For this review, take the finished solid that the model builds, in its own axes (mm). A direction names the side the tool comes from. Round coordinates to 2 decimals unless told otherwise and drop trailing zeros. Order: outer loops, then holes, each group sorted by start corner. A loop starts at its lowest first (then second) coordinate and runs counter-clockwise, first axis right, second up. Notation, with made-up numbers: (-21.75, 44) - (-7.75, 44) arc R11 cw to (-7.75, 57) - close; hole circle Ø10 at (52.25, 86). An arc over 180 degrees is marked (long way). One line per item, written item: value.
```python
from build123d import *

# Parameters (mm, degrees)
AUFSATZ_LINEAR_AUSTRAGEN1_DEPTH = 1.5
SCHNITT_LINEAR_AUSTRAGEN1_REACH = 159.472
SKIZZE2_R                       = 1.3
SKIZZE2_R_2                     = 1
SCHNITT_LINEAR_AUSTRAGEN2_REACH = 159.472
SKIZZE3_W                       = 27
SKIZZE3_H                       = 17.5
SKIZZE4_R                       = 2.5
SKIZZE4_R_2                     = 1.3
AUFSATZ_LINEAR_AUSTRAGEN2_DEPTH = 3
VERRUNDUNG1_R                   = 2
SCHNITT_LINEAR_AUSTRAGEN3_REACH = 159.494
SKIZZE5_W                       = 71.8
SKIZZE5_H                       = 18
VERRUNDUNG2_R                   = 2
SCHNITT_LINEAR_AUSTRAGEN4_REACH = 159.494
SKIZZE6_W                       = 6
SKIZZE6_H                       = 2


with BuildPart() as part:
    # Skizze1 → Aufsatz-Linear austragen1 (new body)
    with BuildSketch(Plane.XY):
        with BuildLine():
            Line((8.4, 0), (113.4, 0))
            ThreePointArc((113.4, 0), (119.339696962, 2.460303038), (121.8, 8.4))
            Line((121.8, 8.4), (121.8, 91.4))
            ThreePointArc((121.8, 91.4), (119.339696962, 97.339696962), (113.4, 99.8))
            Line((113.4, 99.8), (8.4, 99.8))
            ThreePointArc((8.4, 99.8), (2.460303038, 97.339696962), (0, 91.4))
            Line((0, 91.4), (0, 8.4))
            ThreePointArc((0, 8.4), (2.460303038, 2.460303038), (8.4, 0))
        make_face()
    extrude(amount=AUFSATZ_LINEAR_AUSTRAGEN1_DEPTH)

    # Skizze2 → Schnitt-Linear austragen1 (cut, up to next)
    with BuildSketch(Plane.XY.offset(1.5), mode=Mode.PRIVATE) as schnitt_linear_austragen1_sk1:
        with Locations((45.8, 54.2)):
            Circle(SKIZZE2_R)
    schnitt_linear_austragen1_tool1 = extrude(schnitt_linear_austragen1_sk1.sketch, amount=-SCHNITT_LINEAR_AUSTRAGEN1_REACH, mode=Mode.PRIVATE) & part.part
    # Skizze2 → Schnitt-Linear austragen1 (cut, up to next)
    with BuildSketch(Plane.XY.offset(1.5), mode=Mode.PRIVATE) as schnitt_linear_austragen1_sk2:
        with Locations((45.8, 5.2)):
            Circle(SKIZZE2_R)
    schnitt_linear_austragen1_tool2 = extrude(schnitt_linear_austragen1_sk2.sketch, amount=-SCHNITT_LINEAR_AUSTRAGEN1_REACH, mode=Mode.PRIVATE) & part.part
    # Skizze2 → Schnitt-Linear austragen1 (cut, up to next)
    with BuildSketch(Plane.XY.offset(1.5), mode=Mode.PRIVATE) as schnitt_linear_austragen1_sk3:
        with Locations((103.8, 54.2)):
            Circle(SKIZZE2_R)
    schnitt_linear_austragen1_tool3 = extrude(schnitt_linear_austragen1_sk3.sketch, amount=-SCHNITT_LINEAR_AUSTRAGEN1_REACH, mode=Mode.PRIVATE) & part.part
    # Skizze2 → Schnitt-Linear austragen1 (cut, up to next)
    with BuildSketch(Plane.XY.offset(1.5), mode=Mode.PRIVATE) as schnitt_linear_austragen1_sk4:
        with Locations((103.8, 5.2)):
            Circle(SKIZZE2_R)
    schnitt_linear_austragen1_tool4 = extrude(schnitt_linear_austragen1_sk4.sketch, amount=-SCHNITT_LINEAR_AUSTRAGEN1_REACH, mode=Mode.PRIVATE) & part.part
    # Skizze2 → Schnitt-Linear austragen1 (cut, up to next)
    with BuildSketch(Plane.XY.offset(1.5), mode=Mode.PRIVATE) as schnitt_linear_austragen1_sk5:
        with Locations((5.4, 94.4)):
            Circle(SKIZZE2_R_2)
    schnitt_linear_austragen1_tool5 = extrude(schnitt_linear_austragen1_sk5.sketch, amount=-SCHNITT_LINEAR_AUSTRAGEN1_REACH, mode=Mode.PRIVATE) & part.part
    # Skizze2 → Schnitt-Linear austragen1 (cut, up to next)
    with BuildSketch(Plane.XY.offset(1.5), mode=Mode.PRIVATE) as schnitt_linear_austragen1_sk6:
        with Locations((116.4, 94.4)):
            Circle(SKIZZE2_R_2)
    schnitt_linear_austragen1_tool6 = extrude(schnitt_linear_austragen1_sk6.sketch, amount=-SCHNITT_LINEAR_AUSTRAGEN1_REACH, mode=Mode.PRIVATE) & part.part
    # Skizze2 → Schnitt-Linear austragen1 (cut, up to next)
    with BuildSketch(Plane.XY.offset(1.5), mode=Mode.PRIVATE) as schnitt_linear_austragen1_sk7:
        with Locations((116.4, 5.4)):
            Circle(SKIZZE2_R_2)
    schnitt_linear_austragen1_tool7 = extrude(schnitt_linear_austragen1_sk7.sketch, amount=-SCHNITT_LINEAR_AUSTRAGEN1_REACH, mode=Mode.PRIVATE) & part.part
    # Skizze2 → Schnitt-Linear austragen1 (cut, up to next)
    with BuildSketch(Plane.XY.offset(1.5), mode=Mode.PRIVATE) as schnitt_linear_austragen1_sk8:
        with Locations((5.4, 5.4)):
            Circle(SKIZZE2_R_2)
    schnitt_linear_austragen1_tool8 = extrude(schnitt_linear_austragen1_sk8.sketch, amount=-SCHNITT_LINEAR_AUSTRAGEN1_REACH, mode=Mode.PRIVATE) & part.part
    add(schnitt_linear_austragen1_tool1.solids().sort_by_distance((45.8, 54.2, 1.5))[0], mode=Mode.SUBTRACT)
    add(schnitt_linear_austragen1_tool2.solids().sort_by_distance((45.8, 5.2, 1.5))[0], mode=Mode.SUBTRACT)
    add(schnitt_linear_austragen1_tool3.solids().sort_by_distance((103.8, 54.2, 1.5))[0], mode=Mode.SUBTRACT)
    add(schnitt_linear_austragen1_tool4.solids().sort_by_distance((103.8, 5.2, 1.5))[0], mode=Mode.SUBTRACT)
    add(schnitt_linear_austragen1_tool5.solids().sort_by_distance((5.4, 94.4, 1.5))[0], mode=Mode.SUBTRACT)
    add(schnitt_linear_austragen1_tool6.solids().sort_by_distance((116.4, 94.4, 1.5))[0], mode=Mode.SUBTRACT)
    add(schnitt_linear_austragen1_tool7.solids().sort_by_distance((116.4, 5.4, 1.5))[0], mode=Mode.SUBTRACT)
    add(schnitt_linear_austragen1_tool8.solids().sort_by_distance((5.4, 5.4, 1.5))[0], mode=Mode.SUBTRACT)

    # Skizze3 → Schnitt-Linear austragen2 (cut, up to next)
    with BuildSketch(Plane.XY.offset(1.5), mode=Mode.PRIVATE) as schnitt_linear_austragen2_sk1:
        with Locations((100.3, 81.05)):
            Rectangle(SKIZZE3_W, SKIZZE3_H)
    schnitt_linear_austragen2_tool1 = extrude(schnitt_linear_austragen2_sk1.sketch, amount=-SCHNITT_LINEAR_AUSTRAGEN2_REACH, mode=Mode.PRIVATE) & part.part
    add(schnitt_linear_austragen2_tool1.solids().sort_by_distance((100.3, 81.05, 1.5))[0], mode=Mode.SUBTRACT)

    # Skizze4 → Aufsatz-Linear austragen2 (add)
    # profile 1 of 4: a face of its own
    with BuildSketch(Plane(origin=(0, 0, 0), x_dir=(-1, 0, 0), z_dir=(0, 0, -1))):
        with Locations((-103.8, 54.2)):
            Circle(SKIZZE4_R)
        with Locations(Location((-103.8, 54.2, 0), (0, 0, 180))):
            Circle(SKIZZE4_R_2, mode=Mode.SUBTRACT)
    # profile 2 of 4: a face of its own
    with BuildSketch(Plane(origin=(0, 0, 0), x_dir=(-1, 0, 0), z_dir=(0, 0, -1))):
        with Locations((-45.8, 54.2)):
            Circle(SKIZZE4_R)
        with Locations(Location((-45.8, 54.2, 0), (0, 0, 180))):
            Circle(SKIZZE4_R_2, mode=Mode.SUBTRACT)
    # profile 3 of 4: a face of its own
    with BuildSketch(Plane(origin=(0, 0, 0), x_dir=(-1, 0, 0), z_dir=(0, 0, -1))):
        with Locations((-45.8, 5.2)):
            Circle(SKIZZE4_R)
        with Locations(Location((-45.8, 5.2, 0), (0, 0, 180))):
            Circle(SKIZZE4_R_2, mode=Mode.SUBTRACT)
    # profile 4 of 4: a face of its own
    with BuildSketch(Plane(origin=(0, 0, 0), x_dir=(-1, 0, 0), z_dir=(0, 0, -1))):
        with Locations((-103.8, 5.2)):
            Circle(SKIZZE4_R)
        with Locations(Location((-103.8, 5.2, 0), (0, 0, 180))):
            Circle(SKIZZE4_R_2, mode=Mode.SUBTRACT)
    extrude(amount=AUFSATZ_LINEAR_AUSTRAGEN2_DEPTH)

    # Verrundung1
    verrundung1_edges = [part.edges().sort_by_distance(p)[0] for p in [
        (106.3, 54.2, 0),
        (48.3, 54.2, 0),
        (48.3, 5.2, 0),
        (106.3, 5.2, 0),
    ]]
    fillet(verrundung1_edges, radius=VERRUNDUNG1_R)

    # Skizze5 → Schnitt-Linear austragen3 (cut, up to next)
    with BuildSketch(Plane(origin=(0, 0, 0), x_dir=(-1, 0, 0), z_dir=(0, 0, -1)), mode=Mode.PRIVATE) as schnitt_linear_austragen3_sk1:
        with Locations((-45.9, 90.8)):
            Rectangle(SKIZZE5_W, SKIZZE5_H)
    schnitt_linear_austragen3_tool1 = extrude(schnitt_linear_austragen3_sk1.sketch, amount=-SCHNITT_LINEAR_AUSTRAGEN3_REACH, mode=Mode.PRIVATE) & part.part
    add(schnitt_linear_austragen3_tool1.solids().sort_by_distance((45.9, 90.8, 0))[0], mode=Mode.SUBTRACT)

    # Verrundung2
    verrundung2_edges = [part.edges().sort_by_distance(p)[0] for p in [
        (10, 81.8, 0.75),
        (81.8, 81.8, 0.75),
        (10, 99.8, 0.75),
        (81.8, 99.8, 0.75),
    ]]
    fillet(verrundung2_edges, radius=VERRUNDUNG2_R)

    # Skizze6 → Schnitt-Linear austragen4 (cut, up to next)
    with BuildSketch(Plane(origin=(0, 0, 0), x_dir=(-1, 0, 0), z_dir=(0, 0, -1)), mode=Mode.PRIVATE) as schnitt_linear_austragen4_sk1:
        with Locations((-45.9, 77.8)):
            Rectangle(SKIZZE6_W, SKIZZE6_H)
    schnitt_linear_austragen4_tool1 = extrude(schnitt_linear_austragen4_sk1.sketch, amount=-SCHNITT_LINEAR_AUSTRAGEN4_REACH, mode=Mode.PRIVATE) & part.part
    # Skizze6 → Schnitt-Linear austragen4 (cut, up to next)
    with BuildSketch(Plane(origin=(0, 0, 0), x_dir=(-1, 0, 0), z_dir=(0, 0, -1)), mode=Mode.PRIVATE) as schnitt_linear_austragen4_sk2:
        with Locations((-45.9, 65.8)):
            Rectangle(SKIZZE6_W, SKIZZE6_H)
    schnitt_linear_austragen4_tool2 = extrude(schnitt_linear_austragen4_sk2.sketch, amount=-SCHNITT_LINEAR_AUSTRAGEN4_REACH, mode=Mode.PRIVATE) & part.part
    add(schnitt_linear_austragen4_tool1.solids().sort_by_distance((45.9, 77.8, 0))[0], mode=Mode.SUBTRACT)
    add(schnitt_linear_austragen4_tool2.solids().sort_by_distance((45.9, 65.8, 0))[0], mode=Mode.SUBTRACT)


solid = part.part
```
Item 1: Take a section at D-D (x = 85.5). Write out the cut boundary in (y, z), plus the area to 3 significant figures.
Returned:
outline: (0, 0) - (99.8, 0) - (99.8, 1.5) - (0, 1.5) - close
area: 150 mm^2
Item 2: Take a section at C-C (y = 54.2). Write out the cut boundary in (x, z), plus the area to 3 significant figures.
Returned:
outline: (0, 0) - (41.3, 0) arc R2 cw to (43.3, -2) - (43.3, -3) - (44.5, -3) - (44.5, 1.5) - (0, 1.5) - close; (47.1, -3) - (48.3, -3) - (48.3, -2) arc R2 cw to (50.3, 0) - (99.3, 0) arc R2 cw to (101.3, -2) - (101.3, -3) - (102.5, -3) - (102.5, 1.5) - (47.1, 1.5) - close; (105.1, -3) - (106.3, -3) - (106.3, -2) arc R2 cw to (108.3, 0) - (121.8, 0) - (121.8, 1.5) - (105.1, 1.5) - close
area: 193 mm^2
Item 3: The part is to be moulded in two halves that separate along Y. For faces 3 (the cylindrical face through (48.3, 54.3, -2.5)), 4 (the cylindrical face through (119.405, 97.274, 0.74)), 5 (the cylindrical face through (2.395, 2.526, 0.74)), 6 (the cylindrical face through (102.46, 56.31, -2.49)), say which applies: +Y half, -Y half, draft (parallel to the pull), parting line (faces both ways), or undercut.
Returned:
face 3: undercut
face 4: +Y half
face 5: -Y half
face 6: undercut
Item 4: Machinability: for faces 1 (the cylindrical face through (48.3, 5.3, -2.5)), 2 (the cylindrical face through (102.77, 54.99, -0.72)), which of the approach directions +Z, -Z, +X, -X, +Y, -Y give a long, thin tool a straight path to every point of the face, cutting with its end or side? Answer none if there is none.
Returned:
face 1: -Z
face 2: +Z, -Z
Item 5: Take a section at B-B (z = -1). Write out the cut boundary in (x, y).
Returned:
outline: circle Ø5.54 at (45.8, 5.2); circle Ø5.54 at (45.8, 54.2); circle Ø5.54 at (103.8, 5.2); circle Ø5.54 at (103.8, 54.2); hole circle Ø2.6 at (45.8, 5.2); hole circle Ø2.6 at (45.8, 54.2); hole circle Ø2.6 at (103.8, 5.2); hole circle Ø2.6 at (103.8, 54.2)
Item 6: For P1, Ø1.5, axis at x = 94, y = 74, coming from the -Z side; P2, Ø0.8, axis at x = 45, z = 1, coming from the +Y side, all flat-tipped, find the tip position at first contact; note any pin that passes through.
Returned:
P1: through
P2: y = 81.8
Item 7: Wall thickness on line 1 (Y direction, x = 45.8, z = 0.85); line 2 (Y direction, x = 45.8, z = -1.7); line 3 (Y direction, x = 103.8, z = 0.3): over which ranges is each line inside the solid? List them lowest first.
Returned:
line 1: 0 to 3.9, 6.5 to 52.9, 55.5 to 64.8, 66.8 to 76.8, 78.8 to 81.8
line 2: 2.68 to 3.9, 6.5 to 7.72, 51.68 to 52.9, 55.5 to 56.72
line 3: 0 to 3.9, 6.5 to 52.9, 55.5 to 72.3, 89.8 to 99.8
Item 8: Take a section at A-A (x = 103.8). Write out the cut boundary in (y, z), plus the area to 3 significant figures.
Returned:
outline: (0, 0) - (0.7, 0) arc R2 cw to (2.7, -2) - (2.7, -3) - (3.9, -3) - (3.9, 1.5) - (0, 1.5) - close; (6.5, -3) - (7.7, -3) - (7.7, -2) arc R2 cw to (9.7, 0) - (49.7, 0) arc R2 cw to (51.7, -2) - (51.7, -3) - (52.9, -3) - (52.9, 1.5) - (6.5, 1.5) - close; (55.5, -3) - (56.7, -3) - (56.7, -2) arc R2 cw to (58.7, 0) - (72.3, 0) - (72.3, 1.5) - (55.5, 1.5) - close; (89.8, 0) - (99.8, 0) - (99.8, 1.5) - (89.8, 1.5) - close
area: 133 mm^2
